```python
from build123d import *

# Parameters (mm, degrees)
F0_R     = 19.304
F0_R_2   = 1.5875
F1_DEPTH = 3.175
F2_T     = -0.889
F3_DEPTH = 3.176
F4_R     = 18.415
F4_R_2   = 17.907
F5_DEPTH = 0.79375
F6_SIZE  = 0.79374
F7_SIZE  = 0.381


# Not quite as in the source:
# - a fillet or chamfer is up to 0.001 mm smaller than in the source, because OpenCascade refuses the exact size
# - a feature names something its author has since deleted; it is built from what else it names


with BuildPart() as f1:
    # F0 (on Top) → F1 (new body)
    with BuildSketch(Plane.XY):
        Circle(F0_R)
        with Locations((-9.3310908801, -12.8431447857)):
            Circle(F0_R_2, mode=Mode.SUBTRACT)
        with Locations((-15.0980221962, -4.9056447857)):
            Circle(F0_R_2, mode=Mode.SUBTRACT)
        with Locations((-7.8577241059, -7.8577241059)):
            Circle(F0_R_2, mode=Mode.SUBTRACT)
        with Locations((-5.499261314, -3.175)):
            Circle(F0_R_2, mode=Mode.SUBTRACT)
        with Locations((0, -15.875)):
            Circle(F0_R_2, mode=Mode.SUBTRACT)
        with Locations((0, -11.1125)):
            Circle(F0_R_2, mode=Mode.SUBTRACT)
        with Locations((9.3310908801, -12.8431447857)):
            Circle(F0_R_2, mode=Mode.SUBTRACT)
        with Locations((0, -6.35)):
            Circle(F0_R_2, mode=Mode.SUBTRACT)
        with Locations((7.8577241059, -7.8577241059)):
            Circle(F0_R_2, mode=Mode.SUBTRACT)
        with Locations((5.499261314, -3.175)):
            Circle(F0_R_2, mode=Mode.SUBTRACT)
        with Locations((15.0980221962, -4.9056447857)):
            Circle(F0_R_2, mode=Mode.SUBTRACT)
        with Locations((-11.1125, 0)):
            Circle(F0_R_2, mode=Mode.SUBTRACT)
        with Locations((-15.0980221962, 4.9056447857)):
            Circle(F0_R_2, mode=Mode.SUBTRACT)
        with Locations((-5.499261314, 3.175)):
            Circle(F0_R_2, mode=Mode.SUBTRACT)
        with Locations((-7.8577241059, 7.8577241059)):
            Circle(F0_R_2, mode=Mode.SUBTRACT)
        with Locations((-9.3310908801, 12.8431447857)):
            Circle(F0_R_2, mode=Mode.SUBTRACT)
        Circle(F0_R_2, mode=Mode.SUBTRACT)
        with Locations((5.499261314, 3.175)):
            Circle(F0_R_2, mode=Mode.SUBTRACT)
        with Locations((0, 6.35)):
            Circle(F0_R_2, mode=Mode.SUBTRACT)
        with Locations((7.8577241059, 7.8577241059)):
            Circle(F0_R_2, mode=Mode.SUBTRACT)
        with Locations((11.1125, 0)):
            Circle(F0_R_2, mode=Mode.SUBTRACT)
        with Locations((15.0980221962, 4.9056447857)):
            Circle(F0_R_2, mode=Mode.SUBTRACT)
        with Locations((0, 11.1125)):
            Circle(F0_R_2, mode=Mode.SUBTRACT)
        with Locations((9.3310908801, 12.8431447857)):
            Circle(F0_R_2, mode=Mode.SUBTRACT)
        with Locations((0, 15.875)):
            Circle(F0_R_2, mode=Mode.SUBTRACT)
        Circle(F0_R_2)
        with Locations((5.499261314, 3.175)):
            Circle(F0_R_2)
        with Locations((0, 15.875)):
            Circle(F0_R_2)
        with Locations((0, 11.1125)):
            Circle(F0_R_2)
        with Locations((0, 6.35)):
            Circle(F0_R_2)
        with Locations((-9.3310908801, 12.8431447857)):
            Circle(F0_R_2)
        with Locations((-7.8577241059, 7.8577241059)):
            Circle(F0_R_2)
        with Locations((-15.0980221962, 4.9056447857)):
            Circle(F0_R_2)
        with Locations((-11.1125, 0)):
            Circle(F0_R_2)
        with Locations((-5.499261314, 3.175)):
            Circle(F0_R_2)
        with Locations((-15.0980221962, -4.9056447857)):
            Circle(F0_R_2)
        with Locations((-7.8577241059, -7.8577241059)):
            Circle(F0_R_2)
        with Locations((-5.499261314, -3.175)):
            Circle(F0_R_2)
        with Locations((-9.3310908801, -12.8431447857)):
            Circle(F0_R_2)
        with Locations((0, -11.1125)):
            Circle(F0_R_2)
        with Locations((0, -15.875)):
            Circle(F0_R_2)
        with Locations((0, -6.35)):
            Circle(F0_R_2)
        with Locations((7.8577241059, -7.8577241059)):
            Circle(F0_R_2)
        with Locations((9.3310908801, -12.8431447857)):
            Circle(F0_R_2)
        with Locations((15.0980221962, -4.9056447857)):
            Circle(F0_R_2)
        with Locations((11.1125, 0)):
            Circle(F0_R_2)
        with Locations((5.499261314, -3.175)):
            Circle(F0_R_2)
        with Locations((7.8577241059, 7.8577241059)):
            Circle(F0_R_2)
        with Locations((15.0980221962, 4.9056447857)):
            Circle(F0_R_2)
        with Locations((9.3310908801, 12.8431447857)):
            Circle(F0_R_2)
    extrude(amount=F1_DEPTH)

    # F2
    f2_openings = [f1.faces().sort_by_distance(p)[0] for p in [
        (0, 0, 3.175),
    ]]
    offset(amount=F2_T, openings=f2_openings)

    # F0 (on Top) → F3 (cut, through all)
    with BuildSketch(Plane.XY):
        with Locations((0, -6.35)):
            Circle(F0_R_2)
        with Locations((7.8577241059, -7.8577241059)):
            Circle(F0_R_2)
        with Locations((9.3310908801, -12.8431447857)):
            Circle(F0_R_2)
        with Locations((0, -11.1125)):
            Circle(F0_R_2)
        with Locations((0, -15.875)):
            Circle(F0_R_2)
        with Locations((-9.3310908801, -12.8431447857)):
            Circle(F0_R_2)
        with Locations((-7.8577241059, -7.8577241059)):
            Circle(F0_R_2)
        with Locations((-5.499261314, -3.175)):
            Circle(F0_R_2)
        with Locations((-15.0980221962, -4.9056447857)):
            Circle(F0_R_2)
        with Locations((-11.1125, 0)):
            Circle(F0_R_2)
        with Locations((-5.499261314, 3.175)):
            Circle(F0_R_2)
        with Locations((-15.0980221962, 4.9056447857)):
            Circle(F0_R_2)
        with Locations((-9.3310908801, 12.8431447857)):
            Circle(F0_R_2)
        with Locations((-7.8577241059, 7.8577241059)):
            Circle(F0_R_2)
        with Locations((0, 15.875)):
            Circle(F0_R_2)
        with Locations((0, 11.1125)):
            Circle(F0_R_2)
        with Locations((0, 6.35)):
            Circle(F0_R_2)
        with Locations((5.499261314, 3.175)):
            Circle(F0_R_2)
        with Locations((9.3310908801, 12.8431447857)):
            Circle(F0_R_2)
        with Locations((7.8577241059, 7.8577241059)):
            Circle(F0_R_2)
        with Locations((5.499261314, -3.175)):
            Circle(F0_R_2)
        with Locations((15.0980221962, 4.9056447857)):
            Circle(F0_R_2)
        with Locations((15.0980221962, -4.9056447857)):
            Circle(F0_R_2)
        with Locations((11.1125, 0)):
            Circle(F0_R_2)
        Circle(F0_R_2)
    extrude(amount=F3_DEPTH, mode=Mode.SUBTRACT)

    # F4 (on face) → F5 (join)
    with BuildSketch(Plane.XY.offset(3.175)):
        Circle(F4_R)
        Circle(F4_R_2, mode=Mode.SUBTRACT)
    extrude(amount=-F5_DEPTH)

    # F6 (size 0.79375 in the source; OpenCascade refuses exactly that, so slightly less here)
    f6_edges = [f1.edges().sort_by_distance(p)[0] for p in [
        (-17.907, 0, 3.175),
    ]]
    chamfer(f6_edges, length=F6_SIZE)

    # F7
    f7_edges = [f1.edges().sort_by_distance(p)[0] for p in [
        (-18.415, 0, 0.889),
        (18.415, 0, 1.635125),
        (-10.918591, -12.843145, 0.889),
        (-16.685522, -4.905645, 0.889),
        (-9.445224, -7.857724, 0.889),
        (-7.086761, -3.175, 0.889),
        (-1.5875, -15.875, 0.889),
        (-1.5875, -11.1125, 0.889),
        (7.743591, -12.843145, 0.889),
        (-1.5875, -6.35, 0.889),
        (6.270224, -7.857724, 0.889),
        (3.911761, -3.175, 0.889),
        (13.510522, -4.905645, 0.889),
        (-12.7, 0, 0.889),
        (-16.685522, 4.905645, 0.889),
        (-7.086761, 3.175, 0.889),
        (-9.445224, 7.857724, 0.889),
        (-10.918591, 12.843145, 0.889),
        (-1.5875, 0, 0.889),
        (3.911761, 3.175, 0.889),
        (-1.5875, 6.35, 0.889),
        (6.270224, 7.857724, 0.889),
        (9.525, 0, 0.889),
        (13.510522, 4.905645, 0.889),
        (-1.5875, 11.1125, 0.889),
        (-1.5875, 15.875, 0.889),
        (7.743591, 12.843145, 0.889),
    ]]
    chamfer(f7_edges, length=F7_SIZE)


solid = f1.part
```
Model file for the job. Use its own axes, mm. Coordinates: 2 decimals unless noted, no trailing zeros. Answer as a JSON object with one key per item and string values. Group by question number.
(1) Flat gauge pins, fed straight in: pin 1 (1.5 mm diameter, centred on x = -12, y = 0.5, fed in from +Z); pin 2 (4 mm diameter, centred on x = -7.86, y = 7.86, fed in from +Z); pin 3 (6 mm diameter, centred on x = -15, y = 0.5, fed in from +Z). Where does each tip first touch, or does it go through?
(2) Two-plate mould, pull along X, no slides. Class faces 1 (the face through (-13.63, -5.51, 0.25)), 2 (the face through (-15.319, -11.746, 1.565)): released by +X, released by -X, zero draft, split by the parting line, or undercut.
(3) Probe line 1 along X through (y, z) = (-14, 0.5); line 2 along Y through (x, z) = (-17, 0.3); line 3 along X through (y, z) = (3.5, 0.6). List the from-to ranges inside material, lowest first.
(4) Cut at A-A (y = 0). State how many separate pieces and enclosed holes the cut face has, then the cut area to 3 significant figures.
Geometry says:
{
 "1": {"pin 1": "stops at z = 0.69", "pin 2": "stops at z = 0.89", "pin 3": "stops at z = 2.48"},
 "2": {"face 1": "undercut", "face 2": "split by the parting line"},
 "3": {"line 1": "x = -13.29 to -10.42, -8.24 to 8.24, 10.42 to 13.29", "line 2": "y = -9.15 to 9.15", "line 3": "x = -18.98 to -16.02, -14.18 to -7.15, -3.85 to 3.85, 7.15 to 14.18, 16.02 to 18.98"},
 "4": {"separate pieces": "4", "enclosed holes": "0", "area": "29.8 mm^2"}
}
